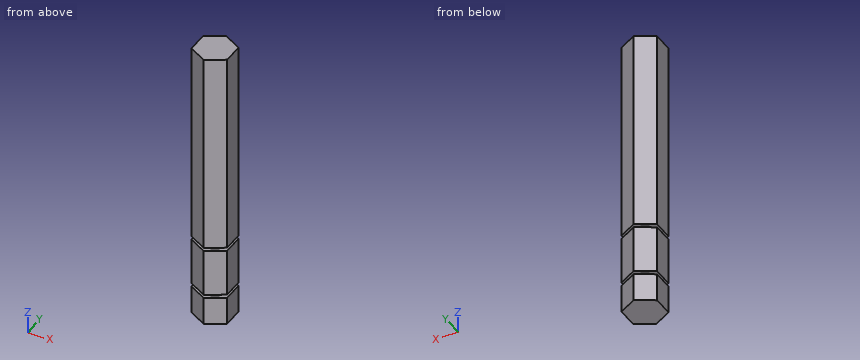
from build123d import *

# Parameters (mm, degrees)
BOSS_EXTRUDE1_DEPTH = 76.2508
SKETCH5_W           = 11.10345239
SKETCH5_H           = 12.145052052
SKETCH5_R           = 3.8481
CUT_EXTRUDE2_DEPTH  = 0.4445
SKETCH6_W           = 10.752068687
SKETCH6_H           = 11.509710708
SKETCH6_R           = 3.8481
CUT_EXTRUDE3_DEPTH  = 0.4445


with BuildPart() as part:
    # Sketch1 → Boss-Extrude1 (new body)
    with BuildSketch(Plane.XY):
        Polygon((0, 5.499261314), (-4.7625, 2.749630657), (-4.7625, -2.749630657), (0, -5.499261314), (4.7625, -2.749630657), (4.7625, 2.749630657), align=None)
    extrude(amount=BOSS_EXTRUDE1_DEPTH)

    # Sketch5 → Cut-Extrude2 (cut, symmetric)
    with BuildSketch(Plane(origin=(0, 0, 21.5138), x_dir=(-1, 0, 0), z_dir=(0, 0, -1))):
        with Locations((-0.378227241, -0.09440181)):
            Rectangle(SKETCH5_W, SKETCH5_H)
        Circle(SKETCH5_R, mode=Mode.SUBTRACT)
    extrude(amount=CUT_EXTRUDE2_DEPTH, both=True, mode=Mode.SUBTRACT)

    # Sketch6 → Cut-Extrude3 (cut, symmetric)
    with BuildSketch(Plane(origin=(0, 0, 7.9502), x_dir=(-1, 0, 0), z_dir=(0, 0, -1))):
        with Locations((-0.265980709, -0.185380495)):
            Rectangle(SKETCH6_W, SKETCH6_H)
        Circle(SKETCH6_R, mode=Mode.SUBTRACT)
    extrude(amount=CUT_EXTRUDE3_DEPTH, both=True, mode=Mode.SUBTRACT)


solid = part.part
Here's how the part is built. I have some questions about the finished solid (model axes, mm). Coordinates: 2 decimals unless noted, no trailing zeros. Write each loop counter-clockwise with the first axis right and the second up, starting at its lowest first coordinate (ties: lowest second). Pieces come first, ordered by that corner, then holes.
Item 1: I want a section at A-A on y = -4.5. Write out the boundary of the cut face in (x, z).
Item 2: Will these pins go through, and if not, where does the flat tip stop? pin 1 (1.5 mm diameter, centred on x = -3.5, z = 61.5, fed in from +Y); pin 2 (2 mm diameter, centred on x = 2.5, z = 25, fed in from -Y).
Item 3: I want a section at C-C on x = -1. Write out the boundary of the cut face in (y, z).
Item 4: If I drill on line 1 (Z direction, x = 1.75, y = -3.75); line 2 (X direction, y = 4, z = 64.5); line 3 (Y direction, x = -2.25, z = 38.5), over which ranges is the centre line in solid material (lowest first)?
Item 5: I want a section at D-D on x = 2. Write out the boundary of the cut face in (y, z), and give its area (3 significant figures).
Item 6: I want a section at B-B on z = 33. Write out the boundary of the cut face in (x, y).
Findings below:
1. outline: (-1.73, 0) - (1.73, 0) - (1.73, 7.51) - (-1.73, 7.51) - close; (-1.73, 8.39) - (1.73, 8.39) - (1.73, 21.07) - (-1.73, 21.07) - close; (-1.73, 21.96) - (1.73, 21.96) - (1.73, 76.25) - (-1.73, 76.25) - close
2. pin 1: stops at y = 3.91
2. pin 2: stops at y = -4.63
3. outline: (-4.92, 0) - (4.92, 0) - (4.92, 7.51) - (3.72, 7.51) - (3.72, 8.39) - (4.92, 8.39) - (4.92, 21.07) - (3.72, 21.07) - (3.72, 21.96) - (4.92, 21.96) - (4.92, 76.25) - (-4.92, 76.25) - (-4.92, 21.96) - (-3.72, 21.96) - (-3.72, 21.07) - (-4.92, 21.07) - (-4.92, 8.39) - (-3.72, 8.39) - (-3.72, 7.51) - (-4.92, 7.51) - close
4. line 1: z = 0 to 7.51, 8.39 to 21.07, 21.96 to 76.25
4. line 2: x = -2.6 to 2.6
4. line 3: y = -4.2 to 4.2
5. outline: (-4.34, 0) - (4.34, 0) - (4.34, 7.51) - (3.29, 7.51) - (3.29, 8.39) - (4.34, 8.39) - (4.34, 21.07) - (3.29, 21.07) - (3.29, 21.96) - (4.34, 21.96) - (4.34, 76.25) - (-4.34, 76.25) - (-4.34, 21.96) - (-3.29, 21.96) - (-3.29, 21.07) - (-4.34, 21.07) - (-4.34, 8.39) - (-3.29, 8.39) - (-3.29, 7.51) - (-4.34, 7.51) - close
5. area: 659 mm2
6. outline: (-4.76, -2.75) - (0, -5.5) - (4.76, -2.75) - (4.76, 2.75) - (0, 5.5) - (-4.76, 2.75) - close
